Job drawing, mm, ordinate dimensions from the low corner. One solid piece. A direction names the side the tool comes from. Give positions to 0.01 mm unless a question says otherwise; leave off trailing zeros. Order: outer loops, then holes, each group sorted by start corner. A loop starts at its lowest first (then second) coordinate and runs counter-clockwise, first axis right, second up. Notation, with made-up numbers: M 29,83.5 L 45,83.5 A13 cw 45,106.5 Z; hole C 51.5,-23.5 d2. An arc over 180 degrees is marked long. One line per question, with ' | ' between items.
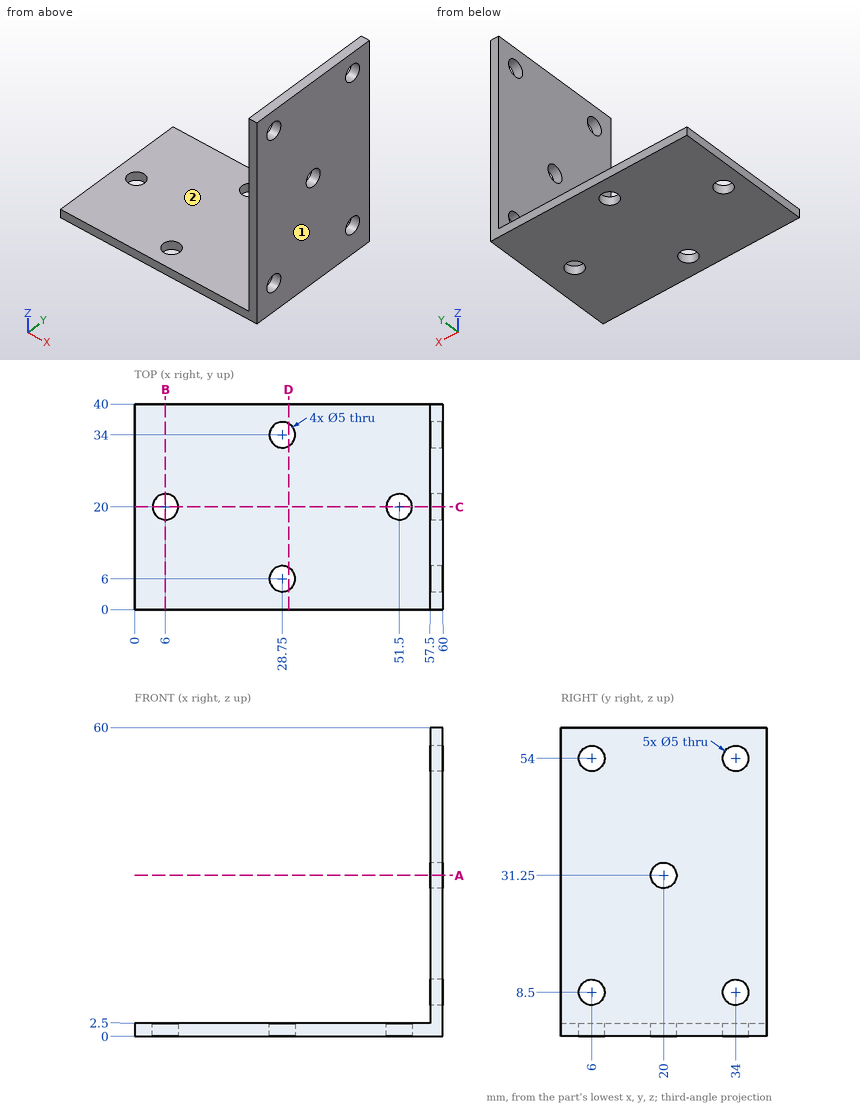
1. Tool access for the marked faces 1 and 2: list every direction of +Z, -Z, +X, -X, +Y, -Y with a clear straight run to the whole face (end or side of a thin tool).
Worked out:
face 1: +Z, -Z, +X, +Y, -Y | face 2: +Z, -X, +Y, -Y
2. Probe L1, parallel to Y at x = 28, z = 1; L2, parallel to Y at x = 51.5, z = 1.4; L3, parallel to X at y = 36, z = 48. List the from-to ranges inside material, lowest first. Write a range as from..to.
Worked out:
L1: y = 0..3.62, 8.38..31.62, 36.38..40 | L2: y = 0..17.5, 22.5..40 | L3: x = 57.5..60
3. Slice it at C-C on y = 20. Give the cut face in (x, z), then the cut area to 3 significant figures.
Worked out:
outline: M 0,0 L 3.5,0 L 3.5,2.5 L 0,2.5 Z; M 8.5,0 L 49,0 L 49,2.5 L 8.5,2.5 Z; M 54,0 L 60,0 L 60,28.75 L 57.5,28.75 L 57.5,2.5 L 54,2.5 Z; M 57.5,33.75 L 60,33.75 L 60,60 L 57.5,60 Z | area: 256 mm2
4. Drop flat-ended pins along their axis: pin 1 (8 mm diameter, centred on x = 18, y = 18, fed in from -Z); pin 2 (4 mm diameter, centred on x = 6, y = 20, fed in from +Z); pin 3 (8 mm diameter, centred on y = 34, z = 8.5, fed in from -X); pin 4 (8 mm diameter, centred on x = 28.75, y = 34, fed in from +Z). Give the stop position or say it passes through.
Worked out:
pin 1: stops at z = 0 | pin 2: passes through | pin 3: stops at x = 57.5 | pin 4: stops at z = 2.5
5. Slice it at A-A on z = 31.25. Give the cut face in (x, y), then the cut area to 3 significant figures.
Worked out:
outline: M 57.5,0 L 60,0 L 60,17.5 L 57.5,17.5 Z; M 57.5,22.5 L 60,22.5 L 60,40 L 57.5,40 Z | area: 87.5 mm2
6. Slice it at B-B on x = 6. Give the cut face in (y, z).
Worked out:
outline: M 0,0 L 17.5,0 L 17.5,2.5 L 0,2.5 Z; M 22.5,0 L 40,0 L 40,2.5 L 22.5,2.5 Z
7. Slice it at D-D on x = 30. Give the cut face in (y, z), then the cut area to 3 significant figures.
Worked out:
outline: M 0,0 L 3.83,0 L 3.83,2.5 L 0,2.5 Z; M 8.17,0 L 31.83,0 L 31.83,2.5 L 8.17,2.5 Z; M 36.17,0 L 40,0 L 40,2.5 L 36.17,2.5 Z | area: 78.3 mm2
